Geometry check sheet. Reference: the model listing, model coordinates, mm. A direction names the side the tool comes from. Coordinates: 2 decimals unless noted, no trailing zeros. Loops run counter-clockwise (first coordinate to the right, second up) from the corner with the lowest first, then second, coordinate; pieces in that order, holes last. Notation, with made-up numbers: (-16.75, 78.5) - (-7.75, 78.5) arc R19 ccw to (-7.75, 111.5) - close; hole circle Ø6 at (46.25, 83). An arc over 180 degrees is marked (long way). One line per item, written item: value.
from build123d import *

# Parameters (mm, degrees)
SKETCH_1_R           = 2.75
EXTRUDE_1_DEPTH      = 1
SKETCH_3_W           = 9.5
SKETCH_3_H           = 9.5
EXTRUDE_2_DEPTH      = 6
SKETCH_12_W          = 9.5
SKETCH_12_H          = 9.5
EXTRUDE_5_DEPTH      = 45
SKETCH_15_W          = 5.9
SKETCH_15_H          = 20.04910328
EXTRUDE_6_DEPTH      = 6
SKETCH_17_R          = 1.8
CUT_EXTRUDE_9_DEPTH  = 5
SKETCH_18_OUTSIDE_W  = 23.92
SKETCH_18_OUTSIDE_H  = 34.47
SKETCH_18_OUTSIDE_R  = 2.75
CUT_EXTRUDE_10_DEPTH = 60
SKETCH_19_R          = 11.5
EXTRUDE_7_DEPTH      = 2
SKETCH_20_R          = 1.25
CUT_EXTRUDE_11_DEPTH = 2
SKETCH_21_R          = 4.5
CUT_EXTRUDE_13_DEPTH = 5.4
SKETCH_22_R          = 2.75
EXTRUDE_8_DEPTH      = 12
CUT_EXTRUDE_START    = -3
SKETCH_24_R          = 2.75
CUT_EXTRUDE_15_DEPTH = 3
SKETCH_25_R          = 1.25
CUT_EXTRUDE_16_DEPTH = 9


with BuildPart() as part:
    # 스케치1 → 보스-돌출1 (new body)
    with BuildSketch(Plane.XY):
        Circle(SKETCH_1_R)
    extrude(amount=EXTRUDE_1_DEPTH)

    # 스케치3 → 보스-돌출2 (add)
    with BuildSketch(Plane(origin=(0, 0, 0), x_dir=(-1, 0, 0), z_dir=(0, 0, -1))):
        Rectangle(SKETCH_3_W, SKETCH_3_H)
    extrude(amount=EXTRUDE_2_DEPTH)

    # 스케치12 → 보스-돌출5 (add)
    with BuildSketch(Plane.XY.offset(1)):
        Rectangle(SKETCH_12_W, SKETCH_12_H)
    extrude(amount=EXTRUDE_5_DEPTH)

    # 스케치15 → 보스-돌출6 (add)
    with BuildSketch(Plane.XY.offset(46)):
        Rectangle(SKETCH_15_W, SKETCH_15_H)
    extrude(amount=EXTRUDE_6_DEPTH)

    # 스케치17 → 컷-돌출9 (cut)
    with BuildSketch(Plane(origin=(0, 4.75, 0), x_dir=(1, 0, 0), z_dir=(0, 1, 0))):
        with Locations(Location((0, -5.1, 0), (0, 0, 180))):
            Circle(SKETCH_17_R)
    extrude(amount=-CUT_EXTRUDE_9_DEPTH, mode=Mode.SUBTRACT)

    # 스케치18 outside → 컷-돌출10 (cut)
    with BuildSketch(Plane(origin=(0, 0, 1), x_dir=(-1, 0, 0), z_dir=(0, 0, -1))):
        Rectangle(SKETCH_18_OUTSIDE_W, SKETCH_18_OUTSIDE_H)
        Circle(SKETCH_18_OUTSIDE_R, mode=Mode.SUBTRACT)
    extrude(amount=-CUT_EXTRUDE_10_DEPTH, mode=Mode.SUBTRACT)

    # 스케치19 → 보스-돌출7 (add)
    with BuildSketch(Plane(origin=(0, 0, -6), x_dir=(-1, 0, 0), z_dir=(0, 0, -1))):
        Circle(SKETCH_19_R)
    extrude(amount=EXTRUDE_7_DEPTH)

    # 스케치20 → 컷-돌출11 (cut)
    with BuildSketch(Plane.XY.offset(-6)):
        with Locations((3.444150891, 8.314915793)):
            Circle(SKETCH_20_R)
        with Locations((8.314915793, 3.444150891)):
            Circle(SKETCH_20_R)
        with Locations((8.314915793, -3.444150891)):
            Circle(SKETCH_20_R)
        with Locations((3.444150891, -8.314915793)):
            Circle(SKETCH_20_R)
        with Locations((-3.444150891, -8.314915793)):
            Circle(SKETCH_20_R)
        with Locations((-8.314915793, -3.444150891)):
            Circle(SKETCH_20_R)
        with Locations((-8.314915793, 3.444150891)):
            Circle(SKETCH_20_R)
        with Locations((-3.444150891, 8.314915793)):
            Circle(SKETCH_20_R)
    extrude(amount=-CUT_EXTRUDE_11_DEPTH, mode=Mode.SUBTRACT)

    # 스케치21 → 컷-돌출13 (cut)
    with BuildSketch(Plane(origin=(0, 0, -8), x_dir=(-1, 0, 0), z_dir=(0, 0, -1))):
        Circle(SKETCH_21_R)
    extrude(amount=-CUT_EXTRUDE_13_DEPTH, mode=Mode.SUBTRACT)

    # 스케치22 → 보스-돌출8 (add)
    with BuildSketch(Plane.XY.offset(52)):
        with Locations(Location((0, 0, 0), (0, 0, 180))):
            Circle(SKETCH_22_R)
    extrude(amount=EXTRUDE_8_DEPTH)

    # 스케치24 → 컷-돌출15 (cut)
    with BuildSketch(Plane.XY.offset(64).offset(CUT_EXTRUDE_START)):
        with Locations(Location((0, 0, 0), (0, 0, 180))):
            Circle(SKETCH_24_R)
    extrude(amount=CUT_EXTRUDE_15_DEPTH, mode=Mode.SUBTRACT)

    # 스케치25 → 컷-돌출16 (cut)
    with BuildSketch(Plane(origin=(0, 2.75, 0), x_dir=(1, 0, 0), z_dir=(0, 1, 0))):
        with Locations(Location((0, -58.6, 0), (0, 0, 270))):
            Circle(SKETCH_25_R)
    extrude(amount=-CUT_EXTRUDE_16_DEPTH, mode=Mode.SUBTRACT)


solid = part.part
(1) Cross-section at B-B on y = -1. Record the cut outline in (x, z).
Reply:
outline: (-11.46, -8) - (-4.39, -8) - (-4.39, -2.6) - (4.39, -2.6) - (4.39, -8) - (11.46, -8) - (11.46, -6) - (4.75, -6) - (4.75, 0) - (2.56, 0) - (2.56, 61) - (-2.56, 61) - (-2.56, 0) - (-4.75, 0) - (-4.75, -6) - (-11.46, -6) - close; hole circle Ø2.5 at (0, 58.6)
(2) Access from +Z, -Z, +X, -X, +Y, -Y to the whole of each face (thin tool, end or side, straight path). Record for faces 1 (the face through (0.59, 4.46, -5.34)), 2 (the face through (2.2, -2, 0)), 3 (the face through (1.428, 1.274, 4.005)).
Reply:
face 1: -Z
face 2: +Z
face 3: +Y
(3) Cross-section at C-C on z = 17. Record the cut outline in (x, y).
Reply:
outline: circle Ø5.5 at (0, 0)
(4) Cross-section at A-A on x = 3.5. Record the cut outline in (y, z).
Reply:
outline: (-10.95, -8) - (-9.56, -8) - (-9.56, -6) - (-10.95, -6) - close; (-7.07, -8) - (-2.83, -8) - (-2.83, -2.6) - (2.83, -2.6) - (2.83, -8) - (7.07, -8) - (7.07, -6) - (4.75, -6) - (4.75, 0) - (-4.75, 0) - (-4.75, -6) - (-7.07, -6) - close; (9.56, -8) - (10.95, -8) - (10.95, -6) - (9.56, -6) - close
(5) Release check for a two-part mould opening along X. For faces 4 (the face through (-4.75, 0, -3)), 5 (the face through (0, -4.75, -3)), 6 (the face through (3.281, 9.554, -6.986)) record: pulls with the +X half, pulls with the -X half, needs draft (parallel to the pull), parting line crosses it, or undercut.
Reply:
face 4: pulls with the -X half
face 5: needs draft
face 6: undercut
(6) Go/stop test with flat-tipped pins: pin 1 Ø12 at (y, z) = (-2, 10) entering from +X; pin 2 Ø10 at (x, z) = (-6, 31) entering from -Y; pin 3 Ø1.8 at (x, z) = (0, -4.5) entering from -Y; pin 4 Ø1.5 at (x, y) = (3.44, -8.31) entering from +Z. Record where each tip stops, or that it passes through.
Reply:
pin 1: x = 2.75
pin 2: y = -2.56
pin 3: y = -4.75
pin 4: through
(7) Material ranges on probe 1 along Z at (x, y) = (0, 1.65); probe 2 along Y at (x, z) = (0, -5.2); probe 3 along Z at (x, y) = (5.75, -7), recorded low to high. Write a range as from..to.
Reply:
probe 1: -2.6..3.3, 6.9..57.35, 59.85..61
probe 2: -4.75..-4.5, 4.5..4.75
probe 3: -8..-6
